Could you check a few things on this drawing? It's one solid part, dimensions in mm from its lowest x, y, z. Round coordinates to 2 decimals unless told otherwise and drop trailing zeros. Write each loop counter-clockwise with the first axis right and the second up, starting at its lowest first coordinate (ties: lowest second). Pieces come first, ordered by that corner, then holes. Notation, with made-up numbers: M 41.25,76.5 L 78.25,76.5 A15 cw 78.25,102.5 Z; hole C 78,64.5 d10. An arc over 180 degrees is marked long. One line per item, written item: value. Start each with the question number.
(1) I want a section at A-A on z = 4.5. Please give me the cut outline in (x, y).
(2) I'm going to push a flat-ended pin straight in: pin 1 Ø2.5 at (x, z) = (4.5, 4.5) entering from -Y. Where does the tip first touch, or does it pass through?
(3) I want a section at B-B on x = 4.5. Please give me the cut outline in (y, z).
(4) I want a section at C-C on y = 0.7. Please give me the cut outline in (x, z).
(5) Thinking about a two-plate mould opening in Z: for the marked faces 1, 2 and 3, which applies, released by +Z, released by -Z, zero draft, split by the parting line, or undercut?
(6) If I drill on L1, parallel to Z at x = 4.5, y = 0.7; L2, parallel to X at y = 0.95, z = 2.75; L3, parallel to X at y = 0.45, z = 3, over which ranges is the centre line in solid material (lowest first)?
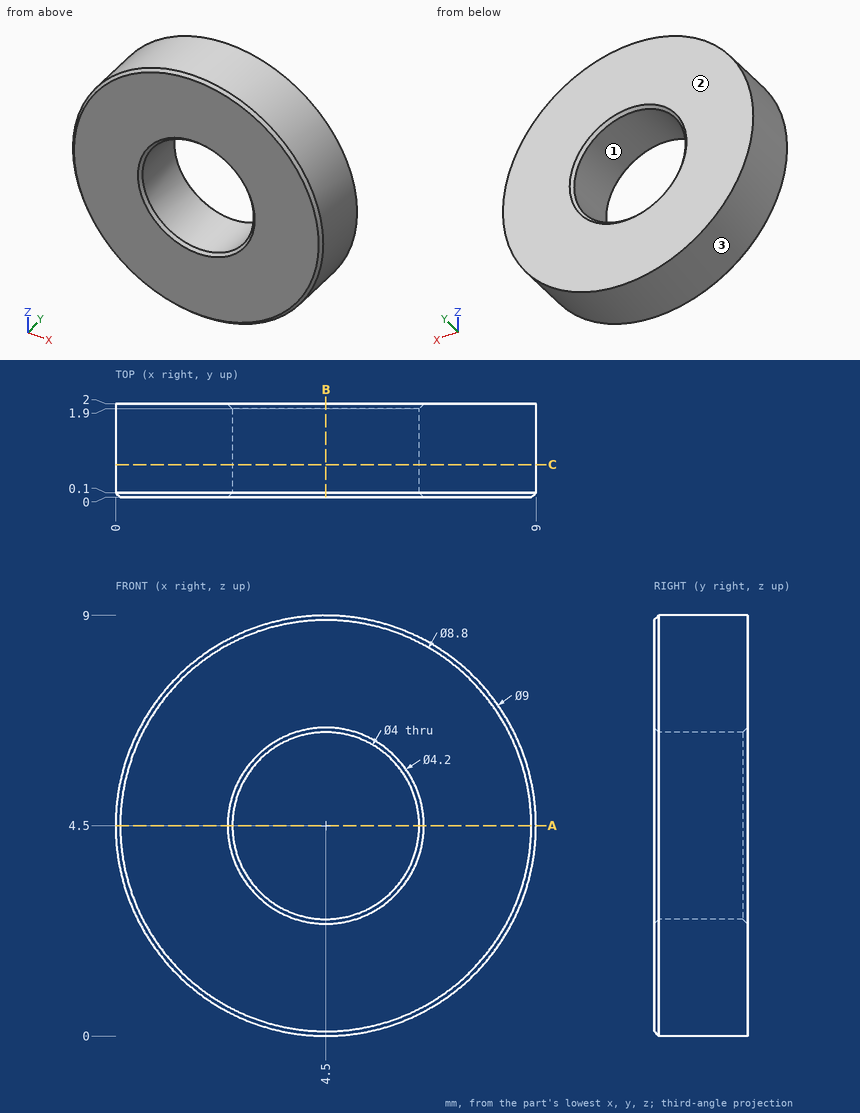
Found:
1. outline: M 0,0.1 L 0.1,0 L 2.4,0 L 2.5,0.1 L 2.5,1.9 L 2.4,2 L 0,2 Z; M 6.5,0.1 L 6.6,0 L 8.9,0 L 9,0.1 L 9,2 L 6.6,2 L 6.5,1.9 Z
2. pin 1: passes through
3. outline: M 0,0.1 L 0.1,0 L 2,0 L 2,2.4 L 1.9,2.5 L 0.1,2.5 L 0,2.4 Z; M 0,6.6 L 0.1,6.5 L 1.9,6.5 L 2,6.6 L 2,9 L 0.1,9 L 0,8.9 Z
4. outline: C 4.5,4.5 d9; hole C 4.5,4.5 d4
5. face 1: undercut
5. face 2: zero draft
5. face 3: split by the parting line
6. L1: z = 0 to 2.5, 6.5 to 9
6. L2: x = 0.35 to 3.53, 5.47 to 8.65
6. L3: x = 0.26 to 3.18, 5.82 to 8.74
